Study the drawing (mm; zero at the part's minimum x, y, z) and answer. A direction names the side the tool comes from. Round coordinates to 2 decimals unless told otherwise and drop trailing zeros. Loops run counter-clockwise (first coordinate to the right, second up) from the corner with the lowest first, then second, coordinate; pieces in that order, holes last. Notation, with made-up numbers: M 87.5,61.5 L 122.5,61.5 A23 cw 122.5,82.5 Z; hole C 41,-37.5 d7. An arc over 180 degrees is marked long. Write each question's results on one line, items separated by ' | '.
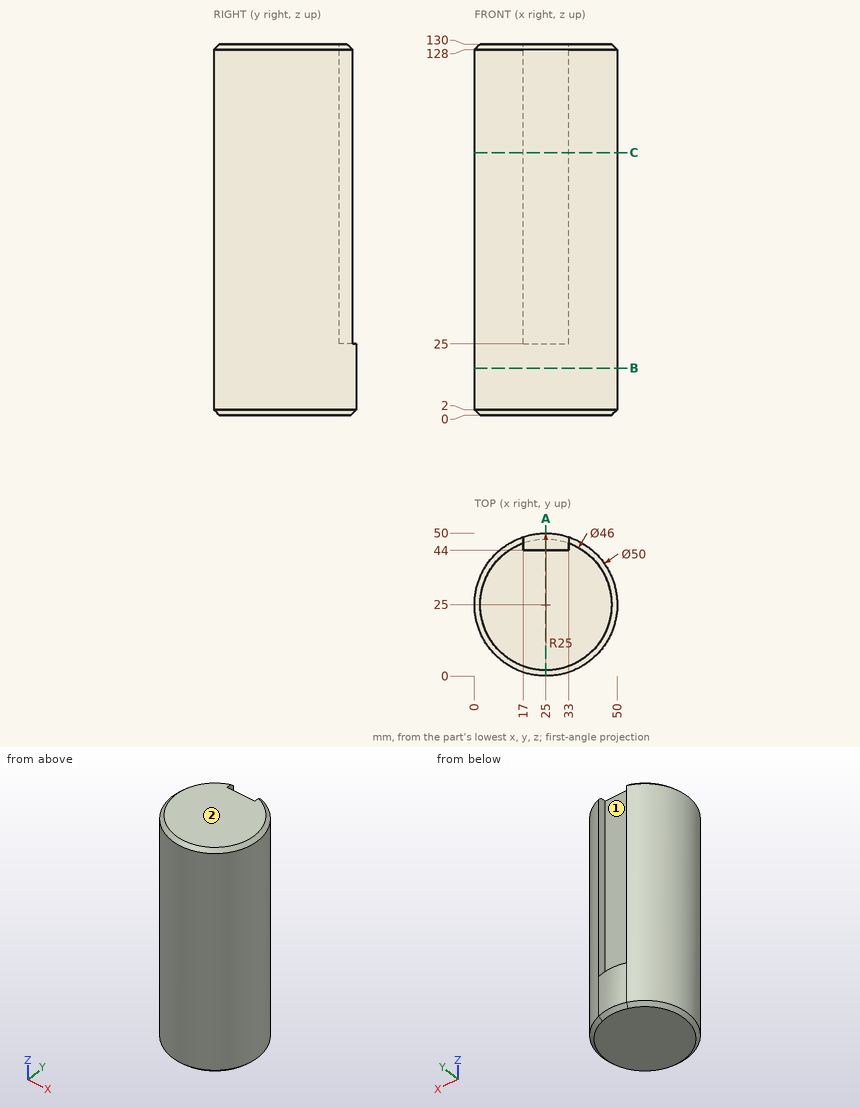
Item 1: The part is cut by section C-C (z = 92). Determine the outline of the cut face in (x, y), plus the area to 3 significant figures.
Outcome:
outline: M 17,44 L 17,48.69 A25 ccw long 33,48.69 L 33,44 Z | area: 1,870 mm2
Item 2: Flat-ended cylindrical pins translate along their axes: pin 1 (4 mm diameter, centred on y = 29, z = 33, fed in from +X); pin 2 (6 mm diameter, centred on y = 26.5, z = 111.5, fed in from +X); pin 3 (5 mm diameter, centred on y = 46, z = 79, fed in from +X). Find the tip coordinate at first contact, or state that the pin passes through.
Outcome:
pin 1: stops at x = 49.92 | pin 2: stops at x = 50 | pin 3: stops at x = 41.82
Item 3: The part is cut by section B-B (z = 16.5). Determine the outline of the cut face in (x, y), plus the area to 3 significant figures.
Outcome:
outline: C 25,25 d50 | area: 1,960 mm2
Item 4: The part is cut by section A-A (x = 25). Determine the outline of the cut face in (y, z).
Outcome:
outline: M 0,2 L 2,0 L 48,0 L 50,2 L 50,25 L 44,25 L 44,130 L 2,130 L 0,128 Z
Item 5: Straight lines are drawn through the part: line 1 (X direction, y = 48, z = 44.5); line 2 (Y direction, x = 22, z = 55.5); line 3 (Y direction, x = 29, z = 99). For each, find the intervals that lie inside material, in ascending order.
Outcome:
line 1: x = 15.2 to 17, 33 to 34.8 | line 2: y = 0.18 to 44 | line 3: y = 0.32 to 44
Item 6: For the marked faces 1 and 2, determine the directions among +Z, -Z, +X, -X, +Y, -Y from which every point of the face is accessible in a straight line to the end or side of a thin tool.
Outcome:
face 1: +Z, +Y | face 2: +Z, +X, -X, +Y, -Y
